Verification items for the finished model (mm, model axes). A direction names the side the tool comes from. Round coordinates to 2 decimals unless told otherwise and drop trailing zeros. Order: outer loops, then holes, each group sorted by start corner. A loop starts at its lowest first (then second) coordinate and runs counter-clockwise, first axis right, second up. Notation, with made-up numbers: (62, -1.5) -> (89, -1.5) arc R27 ccw to (89, 27.5) -> close; hole circle Ø11 at (55.5, 64). An arc over 180 degrees is marked (long way). Put each result on its own line as item: value.
from build123d import *

# Parameters (mm, degrees)
BOSS_EXTRUDE1_DEPTH       = 237.49
BOSS_EXTRUDE2_DEPTH       = 336.55
FILLET1_R                 = 2.54
FILLET2_R                 = 2.54
F_4_CLEARANCE_HOLE3_D     = 2.9464
F_4_CLEARANCE_HOLE3_DEPTH = 25.4
F_4_CLEARANCE_HOLE3_TIP   = 0.885187864
F_4_CLEARANCE_HOLE4_D     = 2.9464
F_4_CLEARANCE_HOLE4_DEPTH = 25.4
F_4_CLEARANCE_HOLE4_TIP   = 0.885187864
F_4_CLEARANCE_HOLE5_D     = 2.9464
F_4_CLEARANCE_HOLE5_DEPTH = 12.7
F_4_CLEARANCE_HOLE5_TIP   = 0.885187864
F_4_CLEARANCE_HOLE6_D     = 2.9464
F_4_CLEARANCE_HOLE6_DEPTH = 12.7
F_4_CLEARANCE_HOLE6_TIP   = 0.885187864


with BuildPart() as part:
    # 3DSketch1 for Loft2 → Loft2 section 0
    with BuildSketch(Plane(origin=(25.14093528, 88.576176245, 12.7), x_dir=(-0.2730484418088959, -0.9620002850445181, 0), z_dir=(0, 0, -1))):
        with BuildLine():
            Line((0, 0), (1.514242104, -0.172182612))
            Line((1.514242104, -0.172182612), (2.214491758, 8.20179449))
            Line((2.214491758, 8.20179449), (18.60742462, 6.462791205))
            Line((18.60742462, 6.462791205), (26.167043779, 33.096731096))
            Line((26.167043779, 33.096731096), (11.304898639, 40.22898334))
            Line((11.304898639, 40.22898334), (15.108293839, 47.722182058))
            Line((15.108293839, 47.722182058), (13.729386407, 48.37117381))
            # circular arc as an exact rational Bezier (weights 1, cos(half-angle), 1)
            Bezier((13.729386407, 48.37117381), (11.15915023, 44.208224795), (9.044543669, 39.796343381), weights=[1, 0.998591281, 1])
            Line((9.044543669, 39.796343381), (24.505322138, 32.380234952))
            Line((24.505322138, 32.380234952), (17.569891716, 7.945427712))
            Line((17.569891716, 7.945427712), (0.518465753, 9.757390103))
            Bezier((0.518465753, 9.757390103), (0, 4.892469572), (0, 0), weights=[1, 0.998591281, 1])
        make_face()
    # Sketch1 for Loft2 → Loft2 section 1
    with BuildSketch(Plane.XY):
        with BuildLine():
            Line((-12.7, 73.846441258), (12.7, 73.846441258))
            Line((12.7, 73.846441258), (16.413015757, 95.436441258))
            Bezier((16.413015757, 95.436441258), (22.196437798, 94.441817026), (27.817431193, 92.756088361), weights=[1, 0.998168879, 1])
            Line((27.817431193, 92.756088361), (27.416130546, 91.417967742))
            Line((27.416130546, 91.417967742), (17.403126873, 93.139989068))
            Line((17.403126873, 93.139989068), (13.843, 72.438989068))
            Line((13.843, 72.438989068), (-13.843, 72.438989068))
            Line((-13.843, 72.438989068), (-17.403126873, 93.139989068))
            Line((-17.403126873, 93.139989068), (-27.416130546, 91.417967742))
            Line((-27.416130546, 91.417967742), (-27.817431193, 92.756088361))
            Bezier((-27.817431193, 92.756088361), (-22.196437798, 94.441817026), (-16.413015757, 95.436441258), weights=[1, 0.998168879, 1])
            Line((-16.413015757, 95.436441258), (-12.7, 73.846441258))
        make_face()
    loft()

    # Sketch1<4> → Boss-Extrude1 (add)
    with BuildSketch(Plane.XY):
        with BuildLine():
            Line((-12.7, 73.846441258), (12.7, 73.846441258))
            Line((12.7, 73.846441258), (16.413015757, 95.436441258))
            ThreePointArc((16.413015757, 95.436441258), (22.155793424, 94.268882586), (27.817431193, 92.756088361))
            Line((27.817431193, 92.756088361), (27.416130546, 91.417967742))
            Line((27.416130546, 91.417967742), (17.403126873, 93.139989068))
            Line((17.403126873, 93.139989068), (13.843, 72.438989068))
            Line((13.843, 72.438989068), (-13.843, 72.438989068))
            Line((-13.843, 72.438989068), (-17.403126873, 93.139989068))
            Line((-17.403126873, 93.139989068), (-27.416130546, 91.417967742))
            Line((-27.416130546, 91.417967742), (-27.817431193, 92.756088361))
            ThreePointArc((-27.817431193, 92.756088361), (-22.155793424, 94.268882586), (-16.413015757, 95.436441258))
            Line((-16.413015757, 95.436441258), (-12.7, 73.846441258))
        make_face()
    extrude(amount=-BOSS_EXTRUDE1_DEPTH)

    # 3DSketch1<4> → Boss-Extrude2 (add)
    with BuildSketch(Plane(origin=(25.14093528, 88.576176245, 12.7), x_dir=(-0.2730484418088959, -0.9620002850445181, 0), z_dir=(0, 0, -1))):
        with BuildLine():
            Line((0, 0), (1.514242104, -0.172182612))
            Line((1.514242104, -0.172182612), (2.214491758, 8.20179449))
            Line((2.214491758, 8.20179449), (18.60742462, 6.462791205))
            Line((18.60742462, 6.462791205), (26.167043779, 33.096731096))
            Line((26.167043779, 33.096731096), (11.304898639, 40.22898334))
            Line((11.304898639, 40.22898334), (15.108293839, 47.722182058))
            Line((15.108293839, 47.722182058), (13.729386407, 48.37117381))
            ThreePointArc((13.729386407, 48.37117381), (11.273137923, 44.14594783), (9.044543669, 39.796343381))
            Line((9.044543669, 39.796343381), (24.505322138, 32.380234952))
            Line((24.505322138, 32.380234952), (17.569891716, 7.945427712))
            Line((17.569891716, 7.945427712), (0.518465753, 9.757390103))
            ThreePointArc((0.518465753, 9.757390103), (0.129707799, 4.885577457), (0, 0))
        make_face()
    extrude(amount=-BOSS_EXTRUDE2_DEPTH)

    # Fillet1
    fillet1_edges = [part.edges().sort_by_distance(p)[0] for p in [
        (-13.843, 72.438989068, -118.745),
        (-13.843, 72.439736297, 6.35),
        (13.843, 72.438989068, -118.745),
        (13.843, 72.439736297, 6.35),
        (-13.843, 72.440483526, 180.975),
        (13.843, 72.440483526, 180.975),
    ]]
    fillet(fillet1_edges, radius=FILLET1_R)

    # Fillet2
    fillet2_edges = [part.edges().sort_by_distance(p)[0] for p in [
        (-12.7, 73.846441258, -118.745),
        (-12.7, 73.844931661, 6.35),
        (12.7, 73.846441258, -118.745),
        (12.7, 73.844931661, 6.35),
        (-12.7, 73.843422063, 180.975),
        (12.7, 73.843422063, 180.975),
    ]]
    fillet(fillet2_edges, radius=FILLET2_R)

    # #4 Clearance Hole3
    with Locations(Plane(origin=(21.064518185, 89.633094885, 0), x_dir=(0.9734791733351508, -0.22877565229436342, 0), z_dir=(0.22877565229436345, 0.9734791733351509, 0))):
        with Locations((0, -336.55), (0, -31.75)):
            Hole(F_4_CLEARANCE_HOLE3_D / 2, depth=F_4_CLEARANCE_HOLE3_DEPTH)
            with Locations((0, 0, -(F_4_CLEARANCE_HOLE3_DEPTH + F_4_CLEARANCE_HOLE3_TIP / 2))):  # 118° drill point
                Cone(0, F_4_CLEARANCE_HOLE3_D / 2, F_4_CLEARANCE_HOLE3_TIP, mode=Mode.SUBTRACT)

    # #4 Clearance Hole4
    with Locations(Plane(origin=(-21.064518185, 89.633094885, 0), x_dir=(0.9734791733351509, 0.2287756522943629, 0), z_dir=(-0.2287756522943629, 0.9734791733351509, 0))):
        with Locations((0, -336.55), (0, -31.75)):
            Hole(F_4_CLEARANCE_HOLE4_D / 2, depth=F_4_CLEARANCE_HOLE4_DEPTH)
            with Locations((0, 0, -(F_4_CLEARANCE_HOLE4_DEPTH + F_4_CLEARANCE_HOLE4_TIP / 2))):  # 118° drill point
                Cone(0, F_4_CLEARANCE_HOLE4_D / 2, F_4_CLEARANCE_HOLE4_TIP, mode=Mode.SUBTRACT)

    # #4 Clearance Hole5
    with Locations(Plane(origin=(-22.154062229, 94.269289448, 0), x_dir=(0.9734791733351509, 0.2287756522943629, 0), z_dir=(-0.2287756522943629, 0.9734791733351509, 0))):
        with Locations((0, 224.79)):
            Hole(F_4_CLEARANCE_HOLE5_D / 2, depth=F_4_CLEARANCE_HOLE5_DEPTH)
            with Locations((0, 0, -(F_4_CLEARANCE_HOLE5_DEPTH + F_4_CLEARANCE_HOLE5_TIP / 2))):  # 118° drill point
                Cone(0, F_4_CLEARANCE_HOLE5_D / 2, F_4_CLEARANCE_HOLE5_TIP, mode=Mode.SUBTRACT)

    # #4 Clearance Hole6
    with Locations(Plane(origin=(22.154062229, 94.269289448, 0), x_dir=(0.9734791733351508, -0.22877565229436342, 0), z_dir=(0.22877565229436345, 0.9734791733351509, 0))):
        with Locations((0, 224.79)):
            Hole(F_4_CLEARANCE_HOLE6_D / 2, depth=F_4_CLEARANCE_HOLE6_DEPTH)
            with Locations((0, 0, -(F_4_CLEARANCE_HOLE6_DEPTH + F_4_CLEARANCE_HOLE6_TIP / 2))):  # 118° drill point
                Cone(0, F_4_CLEARANCE_HOLE6_D / 2, F_4_CLEARANCE_HOLE6_TIP, mode=Mode.SUBTRACT)


solid = part.part
Item 1: Material ranges on L1, parallel to X at y = 80.75, z = 242; L2, parallel to X at y = 75.75, z = -107; L3, parallel to Y at x = -2.5, z = 285.5, recorded low to high. Write a range as [from, to].
Check sheet entries:
L1: x = [-15.28, -13.89], [13.89, 15.28]
L2: x = [-14.41, -13.02], [13.02, 14.41]
L3: y = [72.44, 73.84]
Item 2: Gauge pin test, flat ends, axial feed: pin 1 Ø2 at (y, z) = (91, -172.5) entering from -X; pin 2 Ø4 at (x, z) = (-19.5, 161.5) entering from +Y; pin 3 Ø1.5 at (x, z) = (-0.5, 101) entering from +Y; pin 4 Ø2 at (x, y) = (-13, 88) entering from +Z. Record the tip position at first contact, or that the pin passes through.
Check sheet entries:
pin 1: stops at x = -27.59
pin 2: stops at y = 90.4
pin 3: stops at y = 73.84
pin 4: passes through
Item 3: Tool access check on faces 1 (the flat face through (22.48, 92.267, -117.083)), 2 (the flat face through (0, 72.44, 179)), 3 (the cylindrical face through (22.076, 94.288, -117.083)), 4 (the cylindrical face through (-20.47, 89.77, 178.62)), 5 (the flat face through (14.714, 85.56, -117.083)). Record the directions out of +Z, -Z, +X, -X, +Y, -Y that give a thin tool (end or side, any length) a straight path to the whole face; none if there is none.
Check sheet entries:
face 1: -Z, -Y
face 2: +Z, -Z, +X, -X, -Y
face 3: +Z, -Z, +X, +Y
face 4: +Z, -X, +Y
face 5: +Z, -Z, +Y
Item 4: Section check B-B on z = 158. Record the boundary of the cut face in (x, y) (3 decimals).
Check sheet entries:
outline: (-25.141, 88.576) -> (-24.893, 87.072) -> (-16.646, 88.685) -> (-14.207, 74.549) arc R2.54 ccw to (-11.704, 72.44) -> (11.704, 72.44) arc R2.54 ccw to (14.207, 74.549) -> (16.646, 88.685) -> (24.893, 87.072) -> (25.141, 88.576) arc R92.075 ccw to (15.613, 90.742) -> (13.063, 75.952) arc R2.54 cw to (10.56, 73.843) -> (-10.56, 73.843) arc R2.54 cw to (-13.063, 75.952) -> (-15.613, 90.742) arc R92.075 ccw to start
Item 5: Section check A-A on z = -184.5. Record the boundary of the cut face in (x, y) (1 decimal), then the cut area to 3 significant figures.
Check sheet entries:
outline: (-27.8, 92.8) -> (-27.4, 91.4) -> (-17.4, 93.1) -> (-14.2, 74.5) arc R2.5 ccw to (-11.7, 72.4) -> (11.7, 72.4) arc R2.5 ccw to (14.2, 74.5) -> (17.4, 93.1) -> (27.4, 91.4) -> (27.8, 92.8) arc R96.8 ccw to (16.4, 95.4) -> (13.1, 76) arc R2.5 cw to (10.6, 73.8) -> (-10.6, 73.8) arc R2.5 cw to (-13.1, 76) -> (-16.4, 95.4) arc R96.8 ccw to start
area: 136 mm^2
Item 6: Release check for a two-part mould opening along X. For faces 6 (the cylindrical face through (20.34, 89.8, 178.62)), 7 (the flat face through (-0.52, 73.68, 349.25)), 8 (the flat face through (-22.34, 92.29, -117.08)), 9 (the flat face through (0, 73.846, -117)) record: +X half, -X half, draft (parallel to the pull), parting line (faces both ways), or undercut.
Check sheet entries:
face 6: +X half
face 7: draft
face 8: undercut
face 9: undercut
